Design review of the part built by this model. Coordinates are the model's own, in mm. Face numbers are marked on the shaded views. A direction names the side the tool comes from. Give positions to 0.01 mm unless a question says otherwise; leave off trailing zeros. Loops run counter-clockwise (first coordinate to the right, second up) from the corner with the lowest first, then second, coordinate; pieces in that order, holes last. Notation, with made-up numbers: M -9,-15 L 31,-15 A3 ccw 31,-10 Z; hole C 20,64 d6. An arc over 180 degrees is marked long. Use a Markdown table: item, result. Add a question column.
(1) Add section A-A, the plane z = -30. Give the boundary of the cut face in (x, y).
(2) For the marked faces 4 and 5, list the 3-axis set-ups (+Z, -Z, +X, -X, +Y, -Y) from which the entire face can be reached by the end or side of a thin tool; tool diameter is ignored.
(3) For probe 1 along Z at (x, y) = (12.5, 11); probe 2 along X at (y, z) = (2.5, -30); probe 3 along Y at (x, z) = (56, -45), list the stretches that pass through material, from the lowest coordinate up.
(4) Draft analysis for pull direction Z (two halves, no side actions). For the marked faces 1, 2 and 3, state which applies: pulls with the +Z half, pulls with the -Z half, needs draft (parallel to the pull), parting line crosses it, or undercut.
(5) Add section D-D, the plane x = 20. Give the boundary of the cut face in (y, z).
(6) Add section C-C, the plane z = -54.5. Give the boundary of the cut face in (x, y).
(7) Insertion check: pin 1 Ø12 at (y, z) = (53.5, -50) entering from +X; pin 2 Ø5 at (y, z) = (16, -24.5) entering from -X; pin 3 Ø13 at (x, z) = (49, -27.5) entering from +Y; pin 4 Ø10 at (y, z) = (28.5, -11) entering from +X. Each pin has a flat end and moves straight along its axis. Give the tip position at first contact, or say it passes through.
(8) Add section B-B, the plane y = 10. Give the boundary of the cut face in (x, z), then the cut area to 3 significant figures.
```python
from build123d import *

# Parameters (mm, degrees)
SKETCH1_W           = 68
SKETCH1_H           = 60
BOSS_EXTRUDE1_DEPTH = 8
SKETCH4_W           = 8
SKETCH4_H           = 60
BOSS_EXTRUDE2_DEPTH = 56
SKETCH5_R           = 3.175
CUT_EXTRUDE1_DEPTH  = 8
CUT_EXTRUDE2_DEPTH  = 2
BOSS_EXTRUDE3_DEPTH = 8


with BuildPart() as part:
    # Sketch1 → Boss-Extrude1 (new body)
    with BuildSketch(Plane(origin=(0, 0, 0), x_dir=(1, 0, 0), z_dir=(0, 1, 0))):
        with Locations((34, 30)):
            Rectangle(SKETCH1_W, SKETCH1_H)
    extrude(amount=BOSS_EXTRUDE1_DEPTH)

    # Sketch4 → Boss-Extrude2 (add)
    with BuildSketch(Plane(origin=(0, 8, 0), x_dir=(1, 0, 0), z_dir=(0, 1, 0))):
        with Locations((4, 30)):
            Rectangle(SKETCH4_W, SKETCH4_H)
    extrude(amount=BOSS_EXTRUDE2_DEPTH)

    # Sketch5 → Cut-Extrude1 (cut)
    with BuildSketch(Plane(origin=(0, 8, 0), x_dir=(1, 0, 0), z_dir=(0, 1, 0))):
        with Locations(Location((50.125, 30, 0), (0, 0, 270))):
            Circle(SKETCH5_R)
    extrude(amount=-CUT_EXTRUDE1_DEPTH, mode=Mode.SUBTRACT)

    # Sketch7 → Cut-Extrude2 (cut)
    with BuildSketch(Plane(origin=(0, 8, 0), x_dir=(1, 0, 0), z_dir=(0, 1, 0))):
        Polygon((44.26875, 26.618892486), (50.125, 23.237784972), (55.98125, 26.618892486), (55.98125, 33.381107514), (50.125, 36.762215028), (44.26875, 33.381107514), align=None)
    extrude(amount=-CUT_EXTRUDE2_DEPTH, mode=Mode.SUBTRACT)

    # Sketch8 → Boss-Extrude3 (add)
    with BuildSketch(Plane(origin=(0, 0, -60), x_dir=(-1, 0, 0), z_dir=(0, 0, -1))):
        Polygon((-36, 8), (-8, 8), (-8, 36), align=None)
    boss_extrude3 = extrude(amount=-BOSS_EXTRUDE3_DEPTH)

    # Mirror1: Boss-Extrude3 across plane
    add(boss_extrude3.mirror(Plane(origin=(0, 0, -30), x_dir=(1, 0, 0), z_dir=(0, 0, -1))))


solid = part.part
```
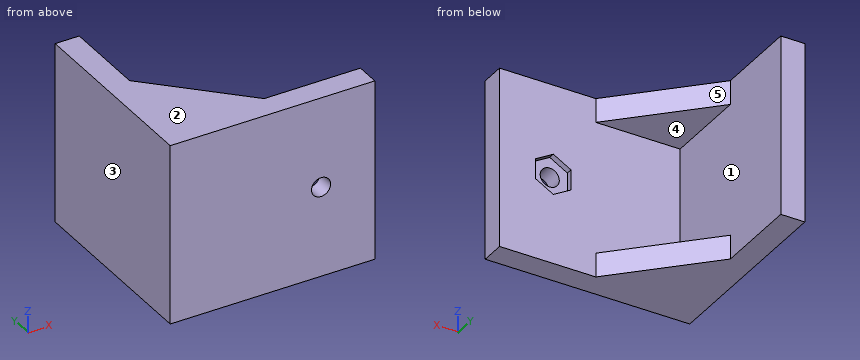
Established:
| question | item | result |
|---|---|---|
| 1 | outline | M 0,0 L 46.95,0 L 46.95,6 L 44.27,6 L 44.27,8 L 8,8 L 8,64 L 0,64 Z; M 53.3,0 L 68,0 L 68,8 L 55.98,8 L 55.98,6 L 53.3,6 Z |
| 2 | face 4 | +X, +Y |
| 2 | face 5 | +Z, -Z, +X, +Y |
| 3 | probe 1 | -60 to -52, -8 to 0 |
| 3 | probe 2 | 0 to 46.95, 53.3 to 68 |
| 3 | probe 3 | 0 to 8 |
| 4 | face 1 | undercut |
| 4 | face 2 | pulls with the +Z half |
| 4 | face 3 | needs draft |
| 5 | outline | M 0,-60 L 24,-60 L 24,-52 L 8,-52 L 8,-8 L 24,-8 L 24,0 L 0,0 Z |
| 6 | outline | M 0,0 L 68,0 L 68,8 L 36,8 L 8,36 L 8,64 L 0,64 Z |
| 7 | pin 1 | x = 8 |
| 7 | pin 2 | x = 0 |
| 7 | pin 3 | y = 8 |
| 7 | pin 4 | x = 19.5 |
| 8 | outline | M 0,-60 L 34,-60 L 34,-52 L 8,-52 L 8,-8 L 34,-8 L 34,0 L 0,0 Z |
| 8 | area | 896 mm^2 |
